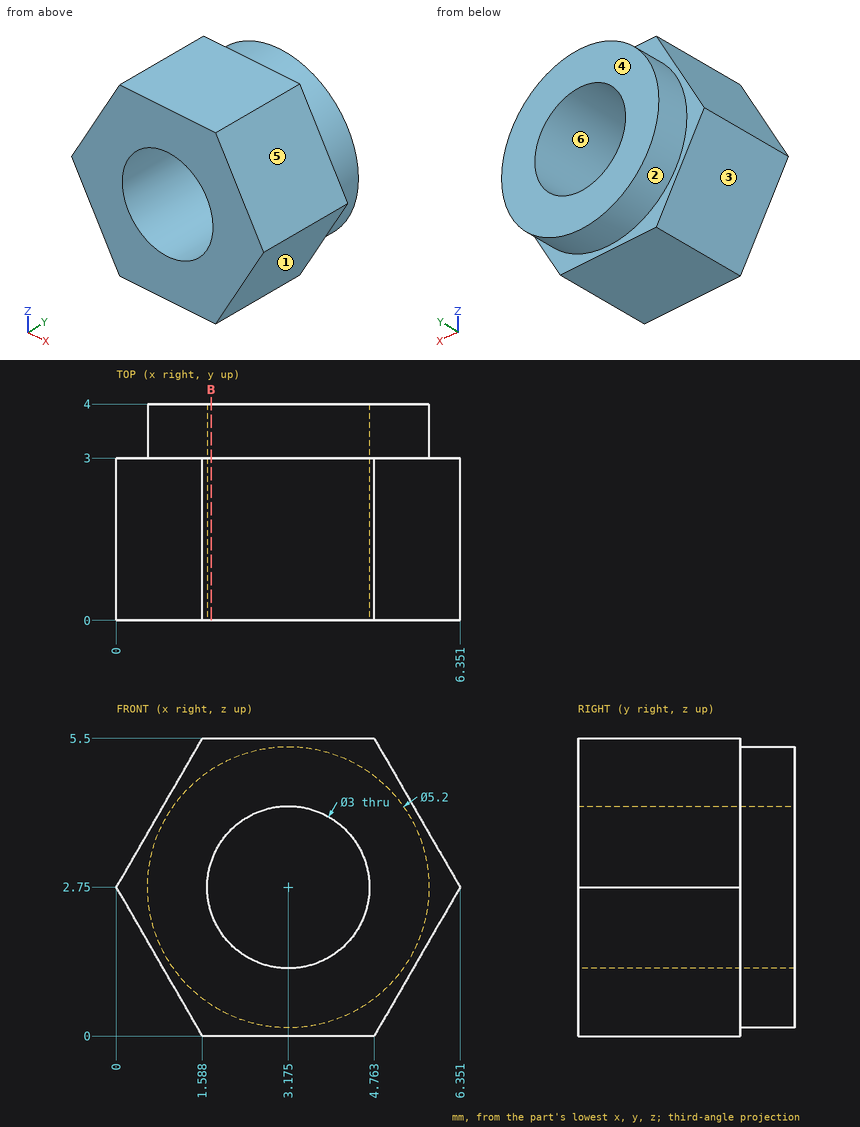
The drawing under review shows one solid part. Ordinate dimensions are in mm from its lowest x, y, z. A direction names the side the tool comes from. Give positions to 0.01 mm unless a question says otherwise; leave off trailing zeros. Write each loop counter-clockwise with the first axis right and the second up, starting at its lowest first coordinate (ties: lowest second). Pieces come first, ordered by that corner, then holes.
1. Draft analysis for pull direction Z (two halves, no side actions). For the marked faces 3, 4, 5 and 6, state which applies: +Z half, -Z half, draft (parallel to the pull), parting line (faces both ways), or undercut.
2. For P1, Ø2.5, axis at x = 3.18, z = 2.75, coming from the +Y side, flat-tipped, find the tip position at first contact; note if it passes through.
3. Add section B-B, the plane x = 1.75. Write out the cut boundary in (y, z) (1 decimal).
4. Wall thickness on L1, parallel to X at y = 3.15, z = 2.75 (1 decimal); L2, parallel to Z at x = 2.75, y = 2.15; L3, parallel to Z at x = 2.5, y = 1.2: over which ranges is each line inside the solid? List them lowest first.
5. Tool access review of the marked faces 1 and 2: name each direction out of +Z, -Z, +X, -X, +Y, -Y from which nothing blocks a thin tool from reaching the whole face with its end or side.
Worked answers:
1. face 3: -Z half
1. face 4: draft
1. face 5: +Z half
1. face 6: undercut
2. P1: passes through
3. outline: (0, 0) - (3, 0) - (3, 0.6) - (4, 0.6) - (4, 2.3) - (0, 2.3) - close; (0, 3.2) - (4, 3.2) - (4, 4.9) - (3, 4.9) - (3, 5.5) - (0, 5.5) - close
4. L1: x = 0.6 to 1.7, 4.7 to 5.8
4. L2: z = 0 to 1.31, 4.19 to 5.5
4. L3: z = 0 to 1.41, 4.09 to 5.5
5. face 1: -Z, +X, +Y, -Y
5. face 2: +Y
